Check sheet for the modelled part. Datum: model origin and axes. Units: mm. A direction names the side the tool comes from. Give positions to 0.01 mm unless a question says otherwise; leave off trailing zeros. Order: outer loops, then holes, each group sorted by start corner. A loop starts at its lowest first (then second) coordinate and runs counter-clockwise, first axis right, second up.
from build123d import *

# Parameters (mm, degrees)
SKETCH_W   = 36
SKETCH_H   = 48
SKETCH_W_2 = 16
SKETCH_H_2 = 24.5
PAD_DEPTH  = 3


with BuildPart() as part:
    # Sketch → Pad (new body)
    with BuildSketch(Plane.XY):
        Rectangle(SKETCH_W, SKETCH_H)
        Polygon((-12.65, 4), (-10.15, 4), (-10.15, -8), (10.15, -8), (10.15, 4), (12.65, 4), (12.65, -17), (10.15, -17), (10.15, -20), (-10.15, -20), (-10.15, -17), (-12.65, -17), align=None, mode=Mode.SUBTRACT)
        with Locations((0, 7.25)):
            Rectangle(SKETCH_W_2, SKETCH_H_2, mode=Mode.SUBTRACT)
    extrude(amount=PAD_DEPTH)


solid = part.part
1) Section check A-A, the plane y = -13. Record the cut outline in (x, z).
Recorded:
outline: (-18, 0) - (-12.65, 0) - (-12.65, 3) - (-18, 3) - close; (12.65, 0) - (18, 0) - (18, 3) - (12.65, 3) - close
2) Material ranges on L1, parallel to Y at x = -1.5, z = 1; L2, parallel to Y at x = -11, z = 1.1; L3, parallel to X at y = 8.5, z = 1.8, recorded low to high.
Recorded:
L1: y = -24 to -20, -8 to -5, 19.5 to 24
L2: y = -24 to -17, 4 to 24
L3: x = -18 to -8, 8 to 18
3) Section check C-C, the plane z = 2.3. Record the cut outline in (x, y).
Recorded:
outline: (-18, -24) - (18, -24) - (18, 24) - (-18, 24) - close; hole (-12.65, -17) - (-10.15, -17) - (-10.15, -20) - (10.15, -20) - (10.15, -17) - (12.65, -17) - (12.65, 4) - (10.15, 4) - (10.15, -8) - (-10.15, -8) - (-10.15, 4) - (-12.65, 4) - close; hole (-8, -5) - (8, -5) - (8, 19.5) - (-8, 19.5) - close
4) Section check D-D, the plane x = 1. Record the cut outline in (y, z).
Recorded:
outline: (-24, 0) - (-20, 0) - (-20, 3) - (-24, 3) - close; (-8, 0) - (-5, 0) - (-5, 3) - (-8, 3) - close; (19.5, 0) - (24, 0) - (24, 3) - (19.5, 3) - close
5) Section check B-B, the plane x = 9. Record the cut outline in (y, z).
Recorded:
outline: (-24, 0) - (-20, 0) - (-20, 3) - (-24, 3) - close; (-8, 0) - (24, 0) - (24, 3) - (-8, 3) - close
6) Draft check along X on faces 3 (the face through (18, 0, 1)), 4 (the face through (-10.15, -2, 1)), 5 (the face through (-8.3, 0.3, 3)). Enter one of: +X half, -X half, draft (parallel to the pull), parting line (faces both ways), or undercut.
Recorded:
face 3: +X half
face 4: undercut
face 5: draft
7) Set-up check for faces 1 (the face through (11, 4, 1)), 2 (the face through (-18, 0, 1)): record each of +Z, -Z, +X, -X, +Y, -Y from which the full face is reachable in a straight line by a thin tool's end or side.
Recorded:
face 1: +Z, -Z
face 2: +Z, -Z, -X, +Y, -Y
